The listing builds one solid part. Answer for the finished solid, in the listing's coordinates (mm). A direction names the side the tool comes from. Coordinates: 2 decimals unless noted, no trailing zeros. Write each loop counter-clockwise with the first axis right and the second up, starting at its lowest first coordinate (ties: lowest second). Pieces come first, ordered by that corner, then holes.
from build123d import *

# Parameters (mm, degrees)
SKETCH1_W           = 100
SKETCH1_H           = 100
BOSS_EXTRUDE1_DEPTH = 50
SHELL1_T            = -5
SKETCH2_W           = 10
SKETCH2_H           = 60
CUT_EXTRUDE1_DEPTH  = 19
SKETCH3_W           = 100
SKETCH3_H           = 100
BOSS_EXTRUDE2_DEPTH = 5


with BuildPart() as part:
    # Sketch1 → Boss-Extrude1 (new body)
    with BuildSketch(Plane.XY):
        Rectangle(SKETCH1_W, SKETCH1_H)
    extrude(amount=BOSS_EXTRUDE1_DEPTH)

    # Shell1
    shell1_openings = [part.faces().sort_by_distance(p)[0] for p in [
        (0, 0, 50),
    ]]
    offset(amount=SHELL1_T, openings=shell1_openings, kind=Kind.INTERSECTION)

    # Sketch2 → Cut-Extrude1 (cut)
    with BuildSketch(Plane(origin=(50, 0, 0), x_dir=(0, 0, -1), z_dir=(1, 0, 0))):
        with Locations((-11.04097714, 0)):
            Rectangle(SKETCH2_W, SKETCH2_H)
    extrude(amount=-CUT_EXTRUDE1_DEPTH, mode=Mode.SUBTRACT)

    # Sketch3 → Boss-Extrude2 (add)
    with BuildSketch(Plane.XY.offset(50)):
        Rectangle(SKETCH3_W, SKETCH3_H)
    extrude(amount=BOSS_EXTRUDE2_DEPTH)


solid = part.part
1. Section A-A on x = 21 is taken. Give the vertices of the cut face in (y, z).
Results found:
outline: (-50, 0) - (50, 0) - (50, 55) - (-50, 55) - close; hole (-45, 5) - (45, 5) - (45, 50) - (-45, 50) - close
2. Section C-C on y = 12.5 is taken. Give the vertices of the cut face in (x, z), then the cut area to 3 significant figures.
Results found:
outline: (-50, 0) - (50, 0) - (50, 6.04) - (45, 6.04) - (45, 5) - (-45, 5) - (-45, 50) - (45, 50) - (45, 16.04) - (50, 16.04) - (50, 55) - (-50, 55) - close
area: 1,400 mm2
3. For a pull along X with two mould halves and no side action, classify faces 1 (the flat face through (50, -1, 27)), 2 (the flat face through (-50, -1, 27)), 3 (the flat face through (45, -1, 32)), 4 (the flat face through (48, 30, 11)) as pulls with the +X half, pulls with the -X half, needs draft (parallel to the pull), parting line crosses it, or undercut.
Results found:
face 1: pulls with the +X half
face 2: pulls with the -X half
face 3: undercut
face 4: needs draft
4. Find the intervals of material crossed by L1, parallel to Y at x = -19, z = 47; L2, parallel to Z at x = 0.5, y = -9, in increasing order.
Results found:
L1: y = -50 to -45, 45 to 50
L2: z = 0 to 5, 50 to 55
5. A tool of negligible diameter and unlimited length cuts with its end or side. For faces 5 (the flat face through (-1, 1, 55)), 6 (the flat face through (-45, -1, 27)), 7 (the flat face through (48, 0, 16.041)), from which of +Z, -Z, +X, -X, +Y, -Y can it reach the whole face along a straight path? Write none if from no direction.
Results found:
face 5: +Z, +X, -X, +Y, -Y
face 6: none
face 7: +X
